Design review of the part built by this model. Coordinates are the model's own, in mm. A direction names the side the tool comes from. Coordinates: 2 decimals unless noted, no trailing zeros. Loops run counter-clockwise (first coordinate to the right, second up) from the corner with the lowest first, then second, coordinate; pieces in that order, holes last. Notation, with made-up numbers: M 40,30 L 66,30 A32 ccw 66,65 Z; hole C 82.25,-34 d3. An arc over 180 degrees is marked long. Put each result on its own line as item: value. Start each with the question number.
(1) Take a section at B-B, the plane z = 0.9. Give the boundary of the cut face in (x, y).
(2) For faces 4 (the flat face through (-1, 0, 0.1)), 5 (the flat face through (0, -7, 1.8)), 6 (the flat face through (-1, 0, 4.4)), 7 (the flat face through (0.3, 0, 2)), 8 (the flat face through (0, -7, 1.4)), list the 3-axis set-ups (+Z, -Z, +X, -X, +Y, -Y) from which the entire face can be reached by the end or side of a thin tool; tool diameter is ignored.
(3) For probe 1 along Z at (x, y) = (2, 0.5); probe 2 along X at (y, z) = (4.5, 4); probe 3 along X at (y, z) = (-3.75, 0.25), list the stretches that pass through material, from the lowest coordinate up. Write a range as [from, to].
(4) The part is to be moulded in two halves that separate along Y. For faces 1 (the flat face through (-2.5, -7, 3.9)), 2 (the flat face through (-0.3, 0, 2)), 3 (the cylindrical face through (0.158, 5.148, 2.218)), say which applies: +Y half, -Y half, draft (parallel to the pull), parting line (faces both ways), or undercut.
(5) Take a section at D-D, the plane y = -8.25. Give the boundary of the cut face in (x, z).
(6) Take a section at A-A, the plane y = -5.5. Give the boundary of the cut face in (x, z).
(7) Clearance check with flat-ended pins moving along their axes: pin 1 (1.8 mm diameter, centred on x = 3, y = -8.5, fed in from -Z); pin 2 (0.5 mm diameter, centred on x = 0, y = -9, fed in from -Z). State where each tip first meets the part, or that it passes through.
(8) Take a section at C-C, the plane y = 0. Give the boundary of the cut face in (x, z).
```python
from build123d import *

# Parameters (mm, degrees)
BOSS_EXTRU_1_DEPTH      = 4.5
ESQUISSE2_W             = 1.6
ESQUISSE2_H             = 0.4
BOSS_EXTRU_2_DEPTH      = 1.5
ESQUISSE3_W             = 1
ESQUISSE3_H             = 0.4
BOSS_EXTRU_3_DEPTH      = 3.5
CHANFREIN1_SIZE         = 0.3
CHANFREIN2_SIZE         = 0.4
ESQUISSE4_R             = 2.5
ENL_V_MAT_EXTRU_1_DEPTH = 0.1
ENL_V_START             = -0.1
ESQUISSE5_R             = 2.5
ENL_V_MAT_EXTRU_2_DEPTH = 0.1
ENL_V_MAT_EXTRU_3_DEPTH = 13.202663644
CONG_1_R                = 1


# Some blends are built 0.0001 mm under size
with BuildPart() as part:
    # Esquisse1 → Boss.-Extru.1 (new body)
    with BuildSketch(Plane.XY):
        with BuildLine():
            Line((-4, -3.243840317), (-4, -5.15))
            Line((-4, -5.15), (4, -5.15))
            Line((4, -5.15), (4, -3.243840317))
            ThreePointArc((4, -3.243840317), (0, 5.15), (-4, -3.243840317))
        make_face()
    extrude(amount=BOSS_EXTRU_1_DEPTH)

    # Esquisse2 → Boss.-Extru.2 (add)
    with BuildSketch(Plane.XZ.offset(5.15)):
        with Locations((-2.5, 4.1)):
            Rectangle(ESQUISSE2_W, ESQUISSE2_H)
        with Locations((2.5, 4.1)):
            Rectangle(ESQUISSE2_W, ESQUISSE2_H)
        with Locations((0, 1.6)):
            Rectangle(ESQUISSE2_W, ESQUISSE2_H)
    extrude(amount=BOSS_EXTRU_2_DEPTH)

    # Esquisse3 → Boss.-Extru.3 (add)
    with BuildSketch(Plane.XZ.offset(6.65)):
        with Locations((-2.5, 4.1)):
            Rectangle(ESQUISSE3_W, ESQUISSE3_H)
        with Locations((2.5, 4.1)):
            Rectangle(ESQUISSE3_W, ESQUISSE3_H)
        with Locations((0, 1.6)):
            Rectangle(ESQUISSE3_W, ESQUISSE3_H)
    extrude(amount=BOSS_EXTRU_3_DEPTH)

    # Chanfrein1
    chanfrein1_edges = [part.edges().sort_by_distance(p)[0] for p in [
        (3, -6.65, 4.1),
        (-2, -6.65, 4.1),
        (0.5, -6.65, 1.6),
        (-0.5, -6.65, 1.6),
        (2, -6.65, 4.1),
        (-3, -6.65, 4.1),
    ]]
    chamfer(chanfrein1_edges, length=CHANFREIN1_SIZE - 0.0001)  # a hair under: the kernel refuses the full size

    # Chanfrein2
    chanfrein2_edges = [part.edges().sort_by_distance(p)[0] for p in [
        (-3, -10.15, 4.1),
        (-2, -10.15, 4.1),
        (2, -10.15, 4.1),
        (3, -10.15, 4.1),
        (-0.5, -10.15, 1.6),
        (0.5, -10.15, 1.6),
    ]]
    chamfer(chanfrein2_edges, length=CHANFREIN2_SIZE)

    # Esquisse4 → Enlèv. mat.-Extru.1 (cut)
    with BuildSketch(Plane(origin=(0, 0, 0), x_dir=(-1, 0, 0), z_dir=(0, 0, -1))):
        Circle(ESQUISSE4_R)
    extrude(amount=-ENL_V_MAT_EXTRU_1_DEPTH, mode=Mode.SUBTRACT)

    # Esquisse5 → Enlèv. mat.-Extru.2 (cut)
    with BuildSketch(Plane.XY.offset(4.5).offset(ENL_V_START)):
        with Locations(Location((0, 0, 0), (0, 0, 180))):
            Circle(ESQUISSE5_R)
    extrude(amount=ENL_V_MAT_EXTRU_2_DEPTH, mode=Mode.SUBTRACT)

    # Esquisse6 → Enlèv. mat.-Extru.3 (cut, through all)
    with BuildSketch(Plane(origin=(0, 0, 0.1), x_dir=(-1, 0, 0), z_dir=(0, 0, -1))):
        Polygon((0, 2), (-0.6, 1.4), (-0.3, 1.4), (-0.3, -2), (0.3, -2), (0.3, 1.4), (0.6, 1.4), align=None)
    extrude(amount=-ENL_V_MAT_EXTRU_3_DEPTH, mode=Mode.SUBTRACT)

    # Congé1
    # the kernel refuses this fillet: 1 mm, written as the material it adds along each edge
    with BuildSketch(Plane(origin=(-4, -3.243840317, 0), x_dir=(0, -1, 0), z_dir=(0, 0, 1))) as cong_1_piece_1:
        with BuildLine():
            CenterArc((0.337011537, -1), CONG_1_R, 90, 35.609116242)
            ThreePointArc((-0.245240797, -0.18699187), (-0.12122038, -0.095332066), (0, 0))
            Line((0, 0), (0.337011537, 0))
        make_face()
    extrude(amount=4.5)
    with BuildSketch(Plane(origin=(4, -3.243840317, 0), x_dir=(0, -1, 0), z_dir=(0, 0, 1))) as cong_1_piece_2:
        with BuildLine():
            CenterArc((0.337011537, 1), CONG_1_R, 234.390883758, 35.609116242)
            ThreePointArc((-0.245240797, 0.18699187), (-0.12122038, 0.095332066), (0, 0))
            Line((0, 0), (0.337011537, 0))
        make_face()
    extrude(amount=4.5)
    # the kernel refuses this fillet: 1 mm, written as the material it takes off along each edge
    with BuildSketch(Plane(origin=(-4, -5.15, -2.5), x_dir=(1, 0, 0), z_dir=(0, 0, 1))) as cong_1_2_piece_1_section:
        with BuildLine():
            CenterArc((CONG_1_R, CONG_1_R), CONG_1_R, 180, 90)
            Line((0, CONG_1_R), (0, 0))
            Line((0, 0), (CONG_1_R, 0))
        make_face()
    cong_1_2_piece_1 = extrude(amount=9.5, mode=Mode.PRIVATE)
    cong_1_2_piece_1 = split(cong_1_2_piece_1, bisect_by=Plane(origin=(-3.3, -5.149735602, 0.7), z_dir=(1, 0, 0)), keep=Keep.TOP, mode=Mode.PRIVATE)
    cong_1_2_piece_1 = split(cong_1_2_piece_1, bisect_by=Plane(origin=(-3.182548732, -5.149735602, 3.9), z_dir=(0, 0, -1)), keep=Keep.TOP, mode=Mode.PRIVATE)
    add(cong_1_2_piece_1, mode=Mode.SUBTRACT)
    with BuildSketch(Plane(origin=(-4, -5.15, -2.5), x_dir=(1, 0, 0), z_dir=(0, 0, 1))) as cong_1_2_piece_2_section:
        with BuildLine():
            CenterArc((CONG_1_R, CONG_1_R), CONG_1_R, 180, 90)
            Line((0, CONG_1_R), (0, 0))
            Line((0, 0), (CONG_1_R, 0))
        make_face()
    cong_1_2_piece_2 = extrude(amount=9.5, mode=Mode.PRIVATE)
    cong_1_2_piece_2 = split(cong_1_2_piece_2, bisect_by=Plane(origin=(-3.3, -4.913833239, 0.7), z_dir=(-1, 0, 0)), keep=Keep.TOP, mode=Mode.PRIVATE)
    cong_1_2_piece_2 = split(cong_1_2_piece_2, bisect_by=Plane(origin=(-3.799145829, -4.913833239, 3.9), z_dir=(0, 0, -1)), keep=Keep.TOP, mode=Mode.PRIVATE)
    add(cong_1_2_piece_2, mode=Mode.SUBTRACT)
    with BuildSketch(Plane(origin=(-4, -5.15, -2.5), x_dir=(1, 0, 0), z_dir=(0, 0, 1))) as cong_1_2_piece_3_section:
        with BuildLine():
            CenterArc((CONG_1_R, CONG_1_R), CONG_1_R, 180, 90)
            Line((0, CONG_1_R), (0, 0))
            Line((0, 0), (CONG_1_R, 0))
        make_face()
    cong_1_2_piece_3 = extrude(amount=9.5, mode=Mode.PRIVATE)
    cong_1_2_piece_3 = split(cong_1_2_piece_3, bisect_by=Plane(origin=(-3.799145829, -4.913833239, 4.3), z_dir=(0, 0, -1)), keep=Keep.TOP, mode=Mode.PRIVATE)
    cong_1_2_piece_3 = split(cong_1_2_piece_3, bisect_by=Plane(origin=(-3.3, -4.913833239, 4.1), z_dir=(-1, 0, 0)), keep=Keep.TOP, mode=Mode.PRIVATE)
    cong_1_2_piece_3 = split(cong_1_2_piece_3, bisect_by=Plane(origin=(-3.799145829, -4.913833239, 3.9), z_dir=(0, 0, 1)), keep=Keep.TOP, mode=Mode.PRIVATE)
    add(cong_1_2_piece_3, mode=Mode.SUBTRACT)
    with BuildSketch(Plane(origin=(-4, -5.15, -2.5), x_dir=(1, 0, 0), z_dir=(0, 0, 1))) as cong_1_2_piece_4_section:
        with BuildLine():
            CenterArc((CONG_1_R, CONG_1_R), CONG_1_R, 180, 90)
            Line((0, CONG_1_R), (0, 0))
            Line((0, 0), (CONG_1_R, 0))
        make_face()
    cong_1_2_piece_4 = extrude(amount=9.5, mode=Mode.PRIVATE)
    cong_1_2_piece_4 = split(cong_1_2_piece_4, bisect_by=Plane(origin=(-3.182548732, -5.149735602, 4.3), z_dir=(0, 0, 1)), keep=Keep.TOP, mode=Mode.PRIVATE)
    cong_1_2_piece_4 = split(cong_1_2_piece_4, bisect_by=Plane(origin=(-3.3, -5.149735602, 5.65), z_dir=(1, 0, 0)), keep=Keep.TOP, mode=Mode.PRIVATE)
    add(cong_1_2_piece_4, mode=Mode.SUBTRACT)
    with BuildSketch(Plane(origin=(-4, -5.15, -2.5), x_dir=(1, 0, 0), z_dir=(0, 0, 1))) as cong_1_2_piece_5_section:
        with BuildLine():
            CenterArc((CONG_1_R, CONG_1_R), CONG_1_R, 180, 90)
            Line((0, CONG_1_R), (0, 0))
            Line((0, 0), (CONG_1_R, 0))
        make_face()
    cong_1_2_piece_5 = extrude(amount=9.5, mode=Mode.PRIVATE)
    cong_1_2_piece_5 = split(cong_1_2_piece_5, bisect_by=Plane(origin=(-3.799145829, -4.913833239, 4.3), z_dir=(0, 0, 1)), keep=Keep.TOP, mode=Mode.PRIVATE)
    cong_1_2_piece_5 = split(cong_1_2_piece_5, bisect_by=Plane(origin=(-3.3, -4.913833239, 5.65), z_dir=(-1, 0, 0)), keep=Keep.TOP, mode=Mode.PRIVATE)
    add(cong_1_2_piece_5, mode=Mode.SUBTRACT)
    with BuildSketch(Plane(origin=(4, -5.15, -2.5), x_dir=(-1, 0, 0), z_dir=(0, 0, 1))) as cong_1_2_piece_6_section:
        with BuildLine():
            CenterArc((CONG_1_R, -CONG_1_R), CONG_1_R, 90, 90)
            Line((0, -CONG_1_R), (0, 0))
            Line((0, 0), (CONG_1_R, 0))
        make_face()
    cong_1_2_piece_6 = extrude(amount=9.5, mode=Mode.PRIVATE)
    cong_1_2_piece_6 = split(cong_1_2_piece_6, bisect_by=Plane(origin=(3.3, -5.149735602, 0.7), z_dir=(-1, 0, 0)), keep=Keep.TOP, mode=Mode.PRIVATE)
    cong_1_2_piece_6 = split(cong_1_2_piece_6, bisect_by=Plane(origin=(3.182548732, -5.149735602, 3.9), z_dir=(0, 0, -1)), keep=Keep.TOP, mode=Mode.PRIVATE)
    add(cong_1_2_piece_6, mode=Mode.SUBTRACT)
    with BuildSketch(Plane(origin=(4, -5.15, -2.5), x_dir=(-1, 0, 0), z_dir=(0, 0, 1))) as cong_1_2_piece_7_section:
        with BuildLine():
            CenterArc((CONG_1_R, -CONG_1_R), CONG_1_R, 90, 90)
            Line((0, -CONG_1_R), (0, 0))
            Line((0, 0), (CONG_1_R, 0))
        make_face()
    cong_1_2_piece_7 = extrude(amount=9.5, mode=Mode.PRIVATE)
    cong_1_2_piece_7 = split(cong_1_2_piece_7, bisect_by=Plane(origin=(3.3, -4.913833239, 0.7), z_dir=(1, 0, 0)), keep=Keep.TOP, mode=Mode.PRIVATE)
    cong_1_2_piece_7 = split(cong_1_2_piece_7, bisect_by=Plane(origin=(3.799145829, -4.913833239, 3.9), z_dir=(0, 0, -1)), keep=Keep.TOP, mode=Mode.PRIVATE)
    add(cong_1_2_piece_7, mode=Mode.SUBTRACT)
    with BuildSketch(Plane(origin=(4, -5.15, -2.5), x_dir=(-1, 0, 0), z_dir=(0, 0, 1))) as cong_1_2_piece_8_section:
        with BuildLine():
            CenterArc((CONG_1_R, -CONG_1_R), CONG_1_R, 90, 90)
            Line((0, -CONG_1_R), (0, 0))
            Line((0, 0), (CONG_1_R, 0))
        make_face()
    cong_1_2_piece_8 = extrude(amount=9.5, mode=Mode.PRIVATE)
    cong_1_2_piece_8 = split(cong_1_2_piece_8, bisect_by=Plane(origin=(3.799145829, -4.913833239, 4.3), z_dir=(0, 0, -1)), keep=Keep.TOP, mode=Mode.PRIVATE)
    cong_1_2_piece_8 = split(cong_1_2_piece_8, bisect_by=Plane(origin=(3.3, -4.913833239, 4.1), z_dir=(1, 0, 0)), keep=Keep.TOP, mode=Mode.PRIVATE)
    cong_1_2_piece_8 = split(cong_1_2_piece_8, bisect_by=Plane(origin=(3.799145829, -4.913833239, 3.9), z_dir=(0, 0, 1)), keep=Keep.TOP, mode=Mode.PRIVATE)
    add(cong_1_2_piece_8, mode=Mode.SUBTRACT)
    with BuildSketch(Plane(origin=(4, -5.15, -2.5), x_dir=(-1, 0, 0), z_dir=(0, 0, 1))) as cong_1_2_piece_9_section:
        with BuildLine():
            CenterArc((CONG_1_R, -CONG_1_R), CONG_1_R, 90, 90)
            Line((0, -CONG_1_R), (0, 0))
            Line((0, 0), (CONG_1_R, 0))
        make_face()
    cong_1_2_piece_9 = extrude(amount=9.5, mode=Mode.PRIVATE)
    cong_1_2_piece_9 = split(cong_1_2_piece_9, bisect_by=Plane(origin=(3.182548732, -5.149735602, 4.3), z_dir=(0, 0, 1)), keep=Keep.TOP, mode=Mode.PRIVATE)
    cong_1_2_piece_9 = split(cong_1_2_piece_9, bisect_by=Plane(origin=(3.3, -5.149735602, 5.65), z_dir=(-1, 0, 0)), keep=Keep.TOP, mode=Mode.PRIVATE)
    add(cong_1_2_piece_9, mode=Mode.SUBTRACT)
    with BuildSketch(Plane(origin=(4, -5.15, -2.5), x_dir=(-1, 0, 0), z_dir=(0, 0, 1))) as cong_1_2_piece_10_section:
        with BuildLine():
            CenterArc((CONG_1_R, -CONG_1_R), CONG_1_R, 90, 90)
            Line((0, -CONG_1_R), (0, 0))
            Line((0, 0), (CONG_1_R, 0))
        make_face()
    cong_1_2_piece_10 = extrude(amount=9.5, mode=Mode.PRIVATE)
    cong_1_2_piece_10 = split(cong_1_2_piece_10, bisect_by=Plane(origin=(3.799145829, -4.913833239, 4.3), z_dir=(0, 0, 1)), keep=Keep.TOP, mode=Mode.PRIVATE)
    cong_1_2_piece_10 = split(cong_1_2_piece_10, bisect_by=Plane(origin=(3.3, -4.913833239, 5.65), z_dir=(1, 0, 0)), keep=Keep.TOP, mode=Mode.PRIVATE)
    add(cong_1_2_piece_10, mode=Mode.SUBTRACT)


solid = part.part
```
Computed values:
1. outline: M -4.19,-3 A1 cw -4,-3.58 L -4,-4.15 A1 ccw -3,-5.15 L 3,-5.15 A1 ccw 4,-4.15 L 4,-3.58 A1 cw 4.19,-3 A5.15 ccw long Z; hole M -0.6,1.4 L -0.3,1.4 L -0.3,-2 L 0.3,-2 L 0.3,1.4 L 0.6,1.4 L 0,2 Z
2. face 4: -Z
2. face 5: +Z, +X, -X, -Y
2. face 6: +Z
2. face 7: +Z, -Z
2. face 8: -Z, +X, -X, -Y
3. probe 1: z = [0.1, 4.4]
3. probe 2: x = [-2.5, 2.5]
3. probe 3: x = [-4, 4]
4. face 1: draft
4. face 2: undercut
4. face 3: parting line
5. outline: M -3,3.9 L -2,3.9 L -2,4.3 L -3,4.3 Z; M -0.5,1.4 L 0.5,1.4 L 0.5,1.8 L -0.5,1.8 Z; M 2,3.9 L 3,3.9 L 3,4.3 L 2,4.3 Z
6. outline: M -3.3,3.9 L -1.7,3.9 L -1.7,4.3 L -3.3,4.3 Z; M -0.8,1.4 L 0.8,1.4 L 0.8,1.8 L -0.8,1.8 Z; M 1.7,3.9 L 3.3,3.9 L 3.3,4.3 L 1.7,4.3 Z
7. pin 1: stops at z = 3.9
7. pin 2: stops at z = 1.4
8. outline: M -5.15,0 L -2.5,0 L -2.5,0.1 L -0.3,0.1 L -0.3,4.4 L -2.5,4.4 L -2.5,4.5 L -5.15,4.5 Z; M 0.3,0.1 L 2.5,0.1 L 2.5,0 L 5.15,0 L 5.15,4.5 L 2.5,4.5 L 2.5,4.4 L 0.3,4.4 Z
